Can you work these out from the model? Positions are in its coordinate system, mm. Face numbers are marked on the shaded views. A direction names the side the tool comes from. Coordinates: 2 decimals unless noted, no trailing zeros. Order: outer loops, then holes, each group sorted by start corner. A loop starts at its lowest first (then second) coordinate and runs counter-clockwise, first axis right, second up. Notation, with made-up numbers: (11, 58.25) -> (22, 58.25) arc R18 ccw to (22, 67.25) -> close; hole circle Ø9 at (30.5, -26). An arc over 180 degrees is marked (long way). Return JSON: item names as keys, results as strings. Group by question number.
1) If we section it at C-C, the plane y = -34: Please give me the cut outline in (x, z).
2) For the marked faces 4 and 5, which set-ups out of +Z, -Z, +X, -X, +Y, -Y let a thin tool reach every point of the face, with its end or its side?
3) Thinking about a two-plate mould opening in Z: for the marked faces 1, 2 and 3, which applies, +Z half, -Z half, draft (parallel to the pull), parting line (faces both ways), or undercut?
4) If I drill on probe 1 along Z at (x, y) = (15, -26); probe 2 along Y at (x, z) = (0, -9.05); probe 3 along Y at (x, z) = (2, -14), over which ranges is the centre line in solid material (lowest first)? Write a range as from..to.
5) For pin 1 (8 mm diameter, centred on x = 4.5, y = 26.5, fed in from +Z); pin 2 (2 mm diameter, centred on x = 0, y = 42, fed in from +Z); pin 3 (1.2 mm diameter, centred on x = 0.5, y = 40, fed in from -Z); pin 4 (0.9 mm diameter, centred on x = 0, y = 42, fed in from +Z), each with a flat end and sliding along its axis, tell me the tip position at first contact or that it passes through.
6) If we section it at B-B, the plane y = 18: Please give me the cut outline in (x, z).
from build123d import *

# Parameters (mm, degrees)
CROQUIS1_R               = 14
MOTOR_DEPTH              = 38
CROQUIS2_R               = 5
SALIENTE_POSTERIOR_DEPTH = 3
BORNES_DEPTH             = 6
CROQUIS4_R               = 0.75
AGUJERO_BORNES_DEPTH     = 24.5
CROQUIS5_R               = 15
CAJA_REDUCTORA_DEPTH     = 24.5
CROQUIS6_R               = 2
BRIDA_DEPTH              = 2.5
CROQUIS7_R               = 6.5
SALIENTE_EJE_DEPTH       = 13.5
CROQUIS8_R               = 3
EJE_DEPTH                = 13.5
CORTE_PLANO_EJE_DEPTH    = 10
CROQUIS10_R              = 2
CORTE_BRIDA_DEPTH        = 10
SALIENTE_EXTRUIR1_START  = 4
CROQUIS11_R              = 14.5
SALIENTE_EXTRUIR1_DEPTH  = 21


with BuildPart() as part:
    # Croquis1 → Motor (new body)
    with BuildSketch(Plane(origin=(0, 0, 0), x_dir=(1, 0, 0), z_dir=(0, 1, 0))):
        Circle(CROQUIS1_R)
    extrude(amount=MOTOR_DEPTH)

    # Croquis2 → Saliente posterior (add)
    with BuildSketch(Plane(origin=(0, 38, 0), x_dir=(1, 0, 0), z_dir=(0, 1, 0))):
        Circle(CROQUIS2_R)
    extrude(amount=SALIENTE_POSTERIOR_DEPTH)

    # Croquis3 → Bornes (add)
    with BuildSketch(Plane(origin=(0, 38, 0), x_dir=(1, 0, 0), z_dir=(0, 1, 0))):
        with BuildLine():
            Line((-2, 9.5), (2, 9.5))
            ThreePointArc((2, 9.5), (2.5, 9), (2, 8.5))
            Line((2, 8.5), (-2, 8.5))
            ThreePointArc((-2, 8.5), (-2.5, 9), (-2, 9.5))
        make_face()
        with BuildLine():
            Line((-2, -9.5), (2, -9.5))
            ThreePointArc((2, -9.5), (2.5, -9), (2, -8.5))
            Line((2, -8.5), (-2, -8.5))
            ThreePointArc((-2, -8.5), (-2.5, -9), (-2, -9.5))
        make_face()
    extrude(amount=BORNES_DEPTH)

    # Croquis4 → Agujero Bornes (cut, through all)
    with BuildSketch(Plane.XY.offset(9.5)):
        with Locations((0, 42)):
            Circle(CROQUIS4_R)
        with BuildLine():
            ThreePointArc((2, 43.866025404), (2.366025404, 43.5), (2.5, 43))
            Line((2.5, 43), (2.5, 44))
            Line((2.5, 44), (2, 44))
            Line((2, 44), (2, 43.866025404))
        make_face()
        with BuildLine():
            ThreePointArc((1.5, 44), (1.758819045, 43.965925826), (2, 43.866025404))
            Line((2, 43.866025404), (2, 44))
            Line((2, 44), (1.5, 44))
        make_face()
        with BuildLine():
            Line((-2, 43.866025404), (-2, 44))
            Line((-2, 44), (-2.5, 44))
            Line((-2.5, 44), (-2.5, 43))
            ThreePointArc((-2.5, 43), (-2.366025404, 43.5), (-2, 43.866025404))
        make_face()
        with BuildLine():
            ThreePointArc((-2, 43.866025404), (-1.758819045, 43.965925826), (-1.5, 44))
            Line((-1.5, 44), (-2, 44))
            Line((-2, 44), (-2, 43.866025404))
        make_face()
    extrude(amount=-AGUJERO_BORNES_DEPTH, mode=Mode.SUBTRACT)

    # Croquis5 → Caja reductora (add)
    with BuildSketch(Plane.XZ):
        Circle(CROQUIS5_R)
    extrude(amount=CAJA_REDUCTORA_DEPTH)

    # Croquis6 → Brida (add)
    with BuildSketch(Plane.XZ.offset(24.5)):
        with BuildLine():
            Line((-15, 20), (15, 20))
            ThreePointArc((15, 20), (18.535533906, 18.535533906), (20, 15))
            Line((20, 15), (20, -15))
            ThreePointArc((20, -15), (18.535533906, -18.535533906), (15, -20))
            Line((15, -20), (-15, -20))
            ThreePointArc((-15, -20), (-18.535533906, -18.535533906), (-20, -15))
            Line((-20, -15), (-20, 15))
            ThreePointArc((-20, 15), (-18.535533906, 18.535533906), (-15, 20))
        make_face()
        with Locations((-15, 15)):
            Circle(CROQUIS6_R, mode=Mode.SUBTRACT)
        with Locations((15, 15)):
            Circle(CROQUIS6_R, mode=Mode.SUBTRACT)
        with Locations((15, -15)):
            Circle(CROQUIS6_R, mode=Mode.SUBTRACT)
        with Locations((-15, -15)):
            Circle(CROQUIS6_R, mode=Mode.SUBTRACT)
    extrude(amount=BRIDA_DEPTH)

    # Croquis7 → Saliente eje (add)
    with BuildSketch(Plane.XZ.offset(27)):
        Circle(CROQUIS7_R)
    extrude(amount=SALIENTE_EJE_DEPTH)

    # Croquis8 → Eje (add)
    with BuildSketch(Plane.XZ.offset(40.5)):
        Circle(CROQUIS8_R)
    extrude(amount=EJE_DEPTH)

    # Croquis9 → Corte Plano eje (cut)
    with BuildSketch(Plane.XZ.offset(54)):
        Polygon((-74.796206056, 2), (-2.236067977, 2), (2.236067977, 2), (74.796206056, 2), (74.796206056, 147.120276157), (-74.796206056, 147.120276157), align=None)
    extrude(amount=-CORTE_PLANO_EJE_DEPTH, mode=Mode.SUBTRACT)

    # Croquis10 → Corte Brida (cut)
    with BuildSketch(Plane(origin=(0, -24.5, 0), x_dir=(1, 0, 0), z_dir=(0, 1, 0))):
        with BuildLine():
            Line((0, 15), (0, 20))
            Line((0, 20), (-15, 20))
            ThreePointArc((-15, 20), (-18.535533906, 18.535533906), (-20, 15))
            Line((-20, 15), (-20, -15))
            ThreePointArc((-20, -15), (-18.535533906, -18.535533906), (-15, -20))
            Line((-15, -20), (0, -20))
            Line((0, -20), (0, -15))
            ThreePointArc((0, -15), (-15, 0), (0, 15))
        make_face()
        with Locations((-15, -15)):
            Circle(CROQUIS10_R, mode=Mode.SUBTRACT)
        with Locations((-15, 15)):
            Circle(CROQUIS10_R, mode=Mode.SUBTRACT)
    extrude(amount=-CORTE_BRIDA_DEPTH, mode=Mode.SUBTRACT)

    # Croquis11 → Saliente-Extruir1 (add)
    with BuildSketch(Plane(origin=(0, 0, 0), x_dir=(1, 0, 0), z_dir=(0, 1, 0)).offset(SALIENTE_EXTRUIR1_START)):
        Circle(CROQUIS11_R)
    extrude(amount=SALIENTE_EXTRUIR1_DEPTH)


solid = part.part
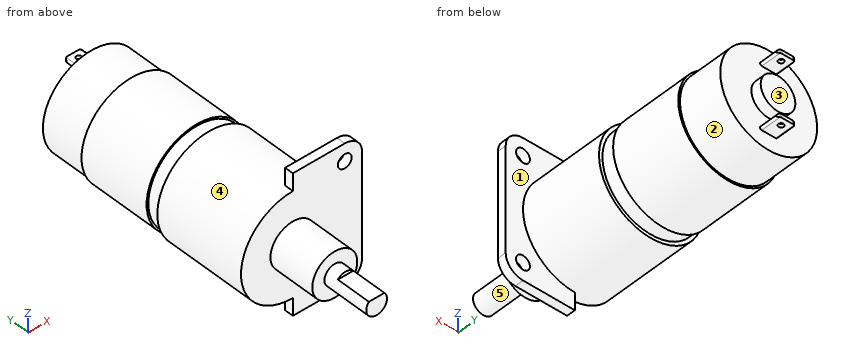
Result sheet:
{
 "1": {"outline": "circle Ø13 at (0, 0)"},
 "2": {"face 4": "+Y", "face 5": "-Y"},
 "3": {"face 1": "draft", "face 2": "parting line", "face 3": "undercut"},
 "4": {"probe 1": "z = -20..-17, -13..13, 17..20", "probe 2": "y = -27..41.25, 42.75..44", "probe 3": "y = -27..0, 4..25"},
 "5": {"pin 1": "stops at z = 14.48", "pin 2": "stops at z = 9.5", "pin 3": "stops at z = -9.5", "pin 4": "passes through"},
 "6": {"outline": "circle Ø29 at (0, 0)"}
}
